Read the model definition and answer for the solid it produces. Units are mm, in the model's axes. A direction names the side the tool comes from. Give positions to 0.01 mm unless a question says otherwise; leave off trailing zeros. Order: outer loops, then holes, each group sorted by start corner. A loop starts at its lowest first (then second) coordinate and runs counter-clockwise, first axis right, second up. Notation, with made-up numbers: (89, -31) - (124, -31) arc R28 ccw to (124, -2) - close; hole circle Ø9 at (33, 36). An arc over 180 degrees is marked (long way). Write item = value, one per line.
```python
from build123d import *

# Parameters (mm, degrees)
F1_DEPTH = 4.7625


with BuildPart() as f1:
    # F0 (on Top) → F1 (new body)
    with BuildSketch(Plane.XY):
        with BuildLine():
            ThreePointArc((-152.4, 63.5), (-147.952155, 63.501619), (-143.51, 63.27672))
            Line((-143.51, 63.27672), (-143.51, 187.182388))
            ThreePointArc((-143.51, 187.182388), (-144.341638, 186.530517), (-145.020427, 185.7207))
            Line((-145.020427, 185.7207), (-247.280253, 34.114273))
            ThreePointArc((-247.280253, 34.114273), (-247.348719, 32.807869), (-246.227376, 32.134098))
            Line((-246.227376, 32.134098), (-220.052506, 32.134098))
            ThreePointArc((-220.052506, 32.134098), (-219.478663, 32.271135), (-219.028659, 32.652674))
            ThreePointArc((-219.028659, 32.652674), (-189.686124, 56.655212), (-152.4, 63.5))
        make_face()
        with BuildLine():
            Line((-98.30838, 20.51779), (-49.596252, 1.226792))
            ThreePointArc((-49.596252, 1.226792), (-52.981384, 31.905787), (-25.70408, 17.4625))
            ThreePointArc((-25.70408, 17.4625), (-26.260302, 13.090239), (-27.893533, 8.996512))
            Line((-27.893533, 8.996512), (-1.59233, 56.445139))
            ThreePointArc((-1.59233, 56.445139), (-0.404525, 59.422396), (0, 62.602222))
            Line((0, 62.602222), (0, 185.42))
            ThreePointArc((0, 185.42), (-0.743949, 187.216051), (-2.54, 187.96))
            Line((-2.54, 187.96), (-140.808916, 187.96))
            ThreePointArc((-140.808916, 187.96), (-142.214311, 187.761728), (-143.51, 187.182388))
            Line((-143.51, 187.182388), (-143.51, 63.27672))
            ThreePointArc((-143.51, 63.27672), (-133.112936, 61.851877), (-122.961928, 59.189894))
            ThreePointArc((-122.961928, 59.189894), (-118.033451, 56.445639), (-114.779625, 51.837664))
            Line((-114.779625, 51.837664), (-104.314477, 26.441552))
            ThreePointArc((-104.314477, 26.441552), (-98.237009, 40.619001), (-84.189692, 34.246517))
            ThreePointArc((-84.189692, 34.246517), (-83.702674, 32.428941), (-83.538674, 30.554409))
            ThreePointArc((-83.538674, 30.554409), (-88.266341, 21.625832), (-98.30838, 20.51779))
        make_face()
        with BuildLine():
            ThreePointArc((-5.08, 60.96), (-9.802601, 55.331824), (-16.165343, 59.005355))
            ThreePointArc((-16.165343, 59.005355), (-11.787399, 66.588176), (-5.08, 60.96))
        make_face(mode=Mode.SUBTRACT)
        with BuildLine():
            ThreePointArc((-49.596252, 1.226792), (-46.439412, 0.30944), (-43.16658, 0))
            ThreePointArc((-43.16658, 0), (-34.303691, 2.416301), (-27.893533, 8.996512))
            ThreePointArc((-27.893533, 8.996512), (-26.260302, 13.090239), (-25.70408, 17.4625))
            ThreePointArc((-25.70408, 17.4625), (-52.981384, 31.905787), (-49.596252, 1.226792))
        make_face()
        with BuildLine():
            ThreePointArc((-104.314477, 26.441552), (-101.91403, 22.868694), (-98.30838, 20.51779))
            ThreePointArc((-98.30838, 20.51779), (-88.266341, 21.625832), (-83.538674, 30.554409))
            ThreePointArc((-83.538674, 30.554409), (-83.702674, 32.428941), (-84.189692, 34.246517))
            ThreePointArc((-84.189692, 34.246517), (-98.237009, 40.619001), (-104.314477, 26.441552))
        make_face()
        with BuildLine():
            ThreePointArc((-88.618674, 30.554409), (-99.96185, 29.56201), (-88.963331, 32.509054))
            ThreePointArc((-88.963331, 32.509054), (-88.705498, 31.546809), (-88.618674, 30.554409))
        make_face(mode=Mode.SUBTRACT)
    extrude(amount=F1_DEPTH)


solid = f1.part
```
1. Section B-B (y = 108.5) is taken. Determine the outline of the cut face in (x, z), and give its area (3 significant figures).
Recorded:
outline = (-197.11, 0) - (0, 0) - (0, 4.76) - (-197.11, 4.76) - close
area = 939 mm^2
2. Determine the mould class of faces 1 (the face through (-0.416, 59.379, 2.348)), 2 (the face through (-133.26, 61.88, 2.35)), 3 (the face through (-233, 32.134, 2)), 4 (the face through (-74.293, 11.007, 2.348)) for opening direction X: +X half, -X half, draft (parallel to the pull), parting line (faces both ways), or undercut.
Recorded:
face_1 = +X half
face_2 = undercut
face_3 = draft
face_4 = -X half
3. For faces 5 (the face through (-14.927, 32.389, 2.348)), 6 (the face through (-190.17, 56.43, 2.35)), determine the directions among +Z, -Z, +X, -X, +Y, -Y from which every point of the face is accessible in a straight line to the end or side of a thin tool.
Recorded:
face_5 = +Z, -Z, +X, -Y
face_6 = +Z, -Z, -Y
4. Section A-A (z = 2.65) is taken. Determine the outline of the cut face in (x, y) (1 decimal).
Recorded:
outline = (-247.3, 34.1) arc R1.3 ccw to (-246.2, 32.1) - (-220.1, 32.1) arc R1.3 ccw to (-219, 32.7) arc R76 cw to (-152.4, 63.5) arc R87.3 cw to (-143.5, 63.3) arc R87.3 cw to (-123, 59.2) arc R12.7 cw to (-114.8, 51.8) - (-104.3, 26.4) arc R10.8 ccw to (-98.3, 20.5) - (-49.6, 1.2) arc R17.5 ccw to (-43.2, 0) arc R17.5 ccw to (-27.9, 9) - (-1.6, 56.4) arc R12.7 ccw to (0, 62.6) - (0, 185.4) arc R2.5 ccw to (-2.5, 188) - (-140.8, 188) arc R5.1 ccw to (-143.5, 187.2) arc R5.1 ccw to (-145, 185.7) - close; hole circle Ø11.4 at (-94.3, 30.6); hole circle Ø11.4 at (-10.8, 61)
5. Section C-C (x = -20) is taken. Determine the outline of the cut face in (y, z).
Recorded:
outline = (23.24, 0) - (187.96, 0) - (187.96, 4.76) - (23.24, 4.76) - close
6. Flat-ended cylindrical pins translate along their axes: pin 1 (1.5 mm diameter, centred on y = 42.5, z = 4, fed in from -X); pin 2 (1.5 mm diameter, centred on y = 141.5, z = 3.5, fed in from -X). Find the tip coordinate at first contact, or state that the pin passes through.
Recorded:
pin_1 = -242.13
pin_2 = -175.35
7. Straight lines are drawn through the part: L1, parallel to X at y = 58, z = 2.3; L2, parallel to Y at x = -106, z = 2.25; L3, parallel to Y at x = -10, z = 1.9. For each, find the intervals that lie inside material, in ascending order. Write a range as [from, to].
Recorded:
L1 = [-231.17, -186.6], [-120.18, -15.68], [-5.91, -0.86]
L2 = [30.53, 187.96]
L3 = [41.28, 55.3], [66.62, 187.96]
